```python
from build123d import *

# Parameters (mm, degrees)
F0_W      = 1244.6
F0_H      = 863.6
F1_DEPTH  = 914.4
F2_W      = 558.8
F2_H      = 355.6
F3_DEPTH  = 889
F4_W      = 558.8
F4_H      = 228.6
F5_DEPTH  = 889
F6_W      = 558.8
F6_H      = 177.8
F7_DEPTH  = 438.15
F8_W      = 558.8
F8_H      = 127
F9_DEPTH  = 438.15
F10_W     = 533.4
F10_H     = 127
F11_DEPTH = 914.4
F12_W     = 533.4
F12_H     = 355.6
F13_DEPTH = 914.4
F14_W     = 50.8
F14_H     = 812.8
F15_DEPTH = 889
F16_W     = 520.7
F16_H     = 279.4
F16_W_2   = 12.7
F17_DEPTH = 889


with BuildPart() as f1:
    # F0 (on Front) → F1 (new body)
    with BuildSketch(Plane.XZ):
        Rectangle(F0_W, F0_H)
    extrude(amount=-F1_DEPTH)

    # F2 (on face) → F3 (cut)
    with BuildSketch(Plane.XZ):
        with Locations((-317.5, -228.6)):
            Rectangle(F2_W, F2_H)
    extrude(amount=-F3_DEPTH, mode=Mode.SUBTRACT)

    # F4 (on face) → F5 (cut)
    with BuildSketch(Plane.XZ):
        with Locations((-317.5, 88.9)):
            Rectangle(F4_W, F4_H)
    extrude(amount=-F5_DEPTH, mode=Mode.SUBTRACT)

    # F6 (on face) → F7 (cut)
    with BuildSketch(Plane.XZ):
        with Locations((-317.5, 317.5)):
            Rectangle(F6_W, F6_H)
    extrude(amount=-F7_DEPTH, mode=Mode.SUBTRACT)

    # F8 (on face) → F9 (cut)
    with BuildSketch(Plane(origin=(0, 914.4, 0), x_dir=(-1, 0, 0), z_dir=(0, 1, 0))):
        with Locations((317.5, 342.9)):
            Rectangle(F8_W, F8_H)
    extrude(amount=-F9_DEPTH, mode=Mode.SUBTRACT)

    # F10 (on face) → F11 (cut)
    with BuildSketch(Plane.XZ):
        with Locations((254, 38.1)):
            Rectangle(F10_W, F10_H)
    extrude(amount=-F11_DEPTH, mode=Mode.SUBTRACT)

    # F12 (on face) → F13 (cut)
    with BuildSketch(Plane.XZ):
        with Locations((254, -228.6)):
            Rectangle(F12_W, F12_H)
    extrude(amount=-F13_DEPTH, mode=Mode.SUBTRACT)

    # F14 (on face) → F15 (cut)
    with BuildSketch(Plane.XZ):
        with Locations((571.5, 0)):
            Rectangle(F14_W, F14_H)
    extrude(amount=-F15_DEPTH, mode=Mode.SUBTRACT)

    # F16 (on face) → F17 (cut)
    with BuildSketch(Plane.XZ):
        with Locations((260.35, 266.7)):
            Rectangle(F16_W, F16_H)
        with Locations((-6.35, 266.7)):
            Rectangle(F16_W_2, F16_H)
    extrude(amount=-F17_DEPTH, mode=Mode.SUBTRACT)


solid = f1.part
```
Verification items for the finished model (mm, model axes). A direction names the side the tool comes from. Coordinates: 2 decimals unless noted, no trailing zeros. Write each loop counter-clockwise with the first axis right and the second up, starting at its lowest first coordinate (ties: lowest second). Pieces come first, ordered by that corner, then holes. Notation, with made-up numbers: (9.5, 89.25) - (23.5, 89.25) arc R7 cw to (23.5, 99.25) - close; hole circle Ø8 at (17.25, 65). An arc over 180 degrees is marked (long way). One line per question, with ' | ' between items. Start each with the question number.
1. Section check C-C (y = 273.5). Count the separate pieces of the cut face and the enclosed holes in it, plus the area to 3 significant figures.
2. Draft check along Z on faces 4 (the flat face through (-9, 451, -431.8)), 5 (the flat face through (-596.9, 216, 316)). Enter one of: released by +Z, released by -Z, zero draft, split by the parting line, or undercut.
3. Material ranges on line 1 along Z through (x, y) = (166, 598); line 2 along X through (y, z) = (304, 359.5); line 3 along X through (y, z) = (694, 115), recorded low to high.
4. Section check A-A (x = 391). Enter the section's corners in (y, z), plus the area to 4 significant figures.
5. Section check D-D (x = -88). Enter the section's corners in (y, z), plus the area to 3 significant figures.
6. Gauge pin test, flat end, axial feed: P1, Ø10, axis at x = -316, z = -231.5, coming from the -Y side. Record the tip position at first contact, or that the pin passes through.
7. Section check B-B (z = 51). Enter the section's corners in (x, y), plus the area to 3 significant figures.
8. Access from +Z, -Z, +X, -X, +Y, -Y to the whole of each face (thin tool, end or side, straight path). Record for faces 1 (the flat face through (250, 451, 101.6)), 2 (the flat face through (-314, 476.25, 344)), 3 (the flat face through (258, 438, 406.4)).
Computed values:
1) separate pieces: 1 | enclosed holes: 7 | area: 201,000 mm²
2) face 4: released by -Z | face 5: undercut
3) line 1: -431.8 to -406.4, -50.8 to -25.4, 101.6 to 127, 406.4 to 431.8 | line 2: -622.3 to -596.9, -38.1 to -12.7, 520.7 to 546.1, 596.9 to 622.3 | line 3: -622.3 to -596.9, -38.1 to 546.1, 596.9 to 622.3
4) outline: (0, -431.8) - (914.4, -431.8) - (914.4, -406.4) - (0, -406.4) - close; (0, -50.8) - (914.4, -50.8) - (914.4, -25.4) - (0, -25.4) - close; (0, 101.6) - (914.4, 101.6) - (914.4, 431.8) - (0, 431.8) - (0, 406.4) - (889, 406.4) - (889, 127) - (0, 127) - close | area: 100,000 mm²
5) outline: (0, -431.8) - (914.4, -431.8) - (914.4, 279.4) - (476.25, 279.4) - (476.25, 406.4) - (914.4, 406.4) - (914.4, 431.8) - (0, 431.8) - (0, 406.4) - (438.15, 406.4) - (438.15, 228.6) - (0, 228.6) - (0, 203.2) - (889, 203.2) - (889, -25.4) - (0, -25.4) - (0, -50.8) - (889, -50.8) - (889, -406.4) - (0, -406.4) - close | area: 137,000 mm²
6) P1: y = 889
7) outline: (-622.3, 0) - (-596.9, 0) - (-596.9, 889) - (-38.1, 889) - (-38.1, 0) - (-12.7, 0) - (-12.7, 914.4) - (-622.3, 914.4) - close; (520.7, 0) - (546.1, 0) - (546.1, 889) - (596.9, 889) - (596.9, 0) - (622.3, 0) - (622.3, 914.4) - (520.7, 914.4) - close | area: 108,000 mm²
8) face 1: +Y, -Y | face 2: +Y | face 3: -Y
